Verification items for the finished model (mm, model axes). A direction names the side the tool comes from. Give positions to 0.01 mm unless a question says otherwise; leave off trailing zeros. Loops run counter-clockwise (first coordinate to the right, second up) from the corner with the lowest first, then second, coordinate; pieces in that order, holes last. Notation, with made-up numbers: (61.5, 6.25) - (115.5, 6.25) arc R16 cw to (115.5, 22.25) - close; hole circle Ø10 at (-5, -39.75). An arc over 180 degrees is marked (long way). Use one line per item in the form item = value.
```python
from build123d import *

# Parameters (mm, degrees)
F0_W          = 20
F0_H          = 22
F0_W_2        = 15.5
F0_H_2        = 15.5
F1_DEPTH      = 20
F2_SIZE       = 2
F3_R          = 1.5
F4_DEPTH      = 7.251
F4_DEPTH_BACK = 25


# Not quite as in the source:
# - a feature names something its author has since deleted; it is built from what else it names


with BuildPart() as f1:
    # F0 (on Front) → F1 (new body)
    with BuildSketch(Plane.XZ):
        with Locations((-38.0418774337, 18.7455339581)):
            Rectangle(F0_W, F0_H)
        with Locations((-38.0418774337, 17.7455339581)):
            Rectangle(F0_W_2, F0_H_2, mode=Mode.SUBTRACT)
        Polygon((-48.0418774337, 29.7455339581), (-28.0418774337, 29.7455339581), (-23.0418774337, 29.7455339581), (-23.0418774337, 34.7455339581), (-53.0418774337, 34.7455339581), (-53.0418774337, 29.7455339581), align=None)
    extrude(amount=F1_DEPTH)

    # F2
    f2_edges = [f1.edges().sort_by_distance(p)[0] for p in [
        (-28.041877, -10, 7.745534),
        (-48.041877, -10, 7.745534),
        (-48.041877, -10, 29.745534),
        (-28.041877, -10, 29.745534),
        (-23.041877, 0, 32.245534),
        (-53.041877, 0, 32.245534),
        (-53.041877, -20, 32.245534),
        (-23.041877, -20, 32.245534),
    ]]
    chamfer(f2_edges, length=F2_SIZE)

    # F3 (on face) → F4 (cut, two sides)
    with BuildSketch(Plane.YZ.offset(-45.7918774337)) as f4_sk:
        with Locations((-10, 17.7455339581)):
            Circle(F3_R)
    extrude(amount=-F4_DEPTH, mode=Mode.SUBTRACT)
    extrude(f4_sk.sketch, amount=F4_DEPTH_BACK, mode=Mode.SUBTRACT)


solid = f1.part
```
1. Tool access check on faces 4 (the flat face through (-25, -10, 29.746)), 5 (the flat face through (-30.292, -10, 16)), 6 (the flat face through (-48.042, -10, 21)). Record the directions out of +Z, -Z, +X, -X, +Y, -Y that give a thin tool (end or side, any length) a straight path to the whole face; none if there is none.
Result set:
face_4 = -Z, +X, +Y, -Y
face_5 = +Y, -Y
face_6 = -Z, -X, +Y, -Y
2. Section check B-B, the plane x = -31. Record the cut outline in (y, z), then the cut area to 3 significant figures.
Result set:
outline = (-20, 7.75) - (0, 7.75) - (0, 10) - (-20, 10) - close; (-20, 25.5) - (0, 25.5) - (0, 34.75) - (-20, 34.75) - close
area = 230 mm²
3. Section check A-A, the plane y = -10. Record the cut outline in (x, z), then the cut area to 3 significant figures.
Result set:
outline = (-53.04, 29.75) - (-50.04, 29.75) - (-48.04, 27.75) - (-48.04, 19.25) - (-45.79, 19.25) - (-45.79, 25.5) - (-30.29, 25.5) - (-30.29, 19.25) - (-28.04, 19.25) - (-28.04, 27.75) - (-26.04, 29.75) - (-23.04, 29.75) - (-23.04, 34.75) - (-53.04, 34.75) - close; (-48.04, 9.75) - (-46.04, 7.75) - (-30.04, 7.75) - (-28.04, 9.75) - (-28.04, 16.25) - (-30.29, 16.25) - (-30.29, 10) - (-45.79, 10) - (-45.79, 16.25) - (-48.04, 16.25) - close
area = 336 mm²
4. Depth check by flat-ended pin: pin 1 Ø4 at (y, z) = (-10, 17.75) entering from +X; pin 2 Ø2.5 at (x, y) = (-51, -9) entering from -Z; pin 3 Ø3 at (x, z) = (-46, 16) entering from +Y; pin 4 Ø2.5 at (x, y) = (-24.5, -7.5) entering from -Z. Enter the tip coordinate at first touch or a pass-through.
Result set:
pin_1 = -28.04
pin_2 = 29.45
pin_3 = 0
pin_4 = 29.75
5. Scan lines: probe 1 along Z at (x, y) = (-36, -10); probe 2 along X at (y, z) = (-15.5, 20.75); probe 3 along Z at (x, y) = (-24.5, -15.5). Record each from-to range of solid material in increasing order.
Result set:
probe_1 = 7.75 to 10, 25.5 to 34.75
probe_2 = -48.04 to -45.79, -30.29 to -28.04
probe_3 = 29.75 to 34.75
6. Draft check along Z on faces 1 (the flat face through (-23.042, -10, 32)), 2 (the flat face through (-45.792, -10, 16)), 3 (the flat face through (-49.056, -9.86, 28.76)). Enter one of: released by +Z, released by -Z, zero draft, split by the parting line, or undercut.
Result set:
face_1 = zero draft
face_2 = undercut
face_3 = released by -Z
7. Section check D-D, the plane y = -7.75. Record the cut outline in (x, z).
Result set:
outline = (-53.04, 29.75) - (-50.04, 29.75) - (-48.04, 27.75) - (-48.04, 9.75) - (-46.04, 7.75) - (-30.04, 7.75) - (-28.04, 9.75) - (-28.04, 27.75) - (-26.04, 29.75) - (-23.04, 29.75) - (-23.04, 34.75) - (-53.04, 34.75) - close; hole (-45.79, 10) - (-30.29, 10) - (-30.29, 25.5) - (-45.79, 25.5) - close
8. Section check C-C, the plane z = 24.5. Record the cut outline in (x, y), then the cut area to 3 significant figures.
Result set:
outline = (-48.04, -20) - (-45.79, -20) - (-45.79, 0) - (-48.04, 0) - close; (-30.29, -20) - (-28.04, -20) - (-28.04, 0) - (-30.29, 0) - close
area = 90.0 mm²
